Can you work these out from the model? Positions are in its coordinate system, mm. Face numbers are marked on the shaded views. A direction names the side the tool comes from. Give positions to 0.01 mm unless a question says otherwise; leave off trailing zeros. Order: outer loops, then holes, each group sorted by start corner. A loop starts at its lowest first (then second) coordinate and runs counter-clockwise, first axis right, second up. Notation, with made-up numbers: (-20.5, 72.25) - (36.5, 72.25) arc R20 cw to (36.5, 90.25) - close; hole circle Ø11 at (-34, 6.5). An arc over 180 degrees is marked (long way). Answer as CSV lines item,"result".
Autodesk Inventor part; units mm, degrees
ref_plane "YZ Plane" through (0, 0, 0) normal (1, 0, 0) x (0, 1, 0)
ref_plane "XZ Plane" through (0, 0, 0) normal (0, 1, 0) x (-1, 0, 0)
ref_plane "XY Plane" through (0, 0, 0) normal (0, 0, 1) x (1, 0, 0)
sketch "Sketch1" plane through (0, 0, 0) normal (0, 0, 1) x (1, 0, 0)
  line L0 (0, 0) -> (0, 10.8481)
  line L1 (0, 10.8481) -> (1.5, 11.25)
  line L2 (1.5, 11.25) -> (1.5, 13.5)
  line L3 (1.5, 13.5) -> (1.7304, 13.5)
  line L4 (2.25, 13.2) -> (2.25, 10.5)
  line L5 (2.25, 10.5) -> (1.5, 10.5)
  line L6 (1.5, 10.5) -> (1.5, 0)
  line L7 (1.5, 0) -> (0, 0)
  line L8 (1.7304, 13.5) -> (2.25, 13.2)
  dimension "Diameter" = 3
  dimension "d1" = 4.5
  dimension "d2" = 3
  dimension "Length" = 10.5
  dimension "d5" = 3
  dimension "d6" = 2.25
  dimension "d7" = 0.3
  dimension "d8" = 30
  dimension "d9" = 15
revolve "Revolution1" add sketch "Sketch1" angle 360 about axis through (0, 0, 0) along (0, 1, 0)
sketch "Sketch2" plane through (0, 13.5, 0) normal (0, 1, 0) x (1, 0, 0)
  circle A0 centre (0, 0) radius 1.5
  line L0 (0, -1.299) -> (-1.125, -0.6495)
  line L1 (-1.125, -0.6495) -> (-1.125, 0.6495)
  line L2 (-1.125, 0.6495) -> (0, 1.299)
  line L3 (0, 1.299) -> (1.125, 0.6495)
  line L4 (1.125, 0.6495) -> (1.125, -0.6495)
  line L5 (1.125, -0.6495) -> (0, -1.299)
  dimension "d14" = 2.25
extrude "Extrusion1" add sketch "Sketch2" against normal up to next
thread "Thread2"
chamfer "Chamfer2" distance 0.2 angle 45 1 edges at (-1.5, 0, 0)
fillet "Fillet1" radius 0.1 1 edges at (-1.5, 10.5, 0)
equation "\"d1\" = 1.5 * Diameter"
equation "\"d2\" = Diameter"
equation "\"d5\" = Diameter"
equation "\"d6\" = 0.75 * Diameter"
equation "\"d7\" = 0.1 * Diameter"
equation "\"d14\" = 0.75 * Diameter"
properties part number "Hex Socket Screw"
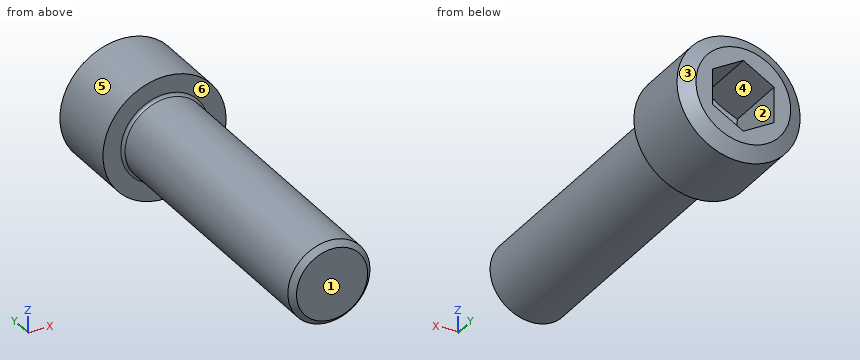
1) If we mould it in two halves opening along Z, with no side actions, what happens to the marked faces 1, 2 and 3? For each: +Z half, -Z half, draft (parallel to the pull), parting line (faces both ways), or undercut.
Answer block:
face 1,"draft"
face 2,"undercut"
face 3,"parting line"
2) I want a section at A-A on y = 3.5. Write out the boundary of the cut face in (x, z), plus the area to 3 significant figures.
Answer block:
outline,"circle Ø3 at (0, 0)"
area,"7.07 mm2"
3) I'm going to push a flat-ended pin straight in: P1, Ø2, axis at y = 4.5, z = 0.5, coming from the -X side. Where does the tip first touch, or does it pass through?
Answer block:
P1,"x = -1.5"
4) Which directions (+Z, -Z, +X, -X, +Y, -Y) give clear straight access to the entire face, cutting with the end or side of a thin tool? Please do the marked faces 4, 5 and 6.
Answer block:
face 4,"+Y"
face 5,"+Y, -Y"
face 6,"-Y"
5) I need wall thicknesses on line 1 along X through (y, z) = (11.5, -0.05) (3 decimals); line 2 along X through (y, z) = (2.75, 0.75); line 3 along Z through (x, y) = (-0.3, 13). Which ranges of each line are inside material? Lowest first, please. Write a range as [from, to].
Answer block:
line 1,"[-2.249, -1.125], [1.125, 2.249]"
line 2,"[-1.3, 1.3]"
line 3,"[-2.23, -1.13], [1.13, 2.23]"
